Read the model definition and answer for the solid it produces. Units are mm, in the model's axes. Coordinates: 2 decimals unless noted, no trailing zeros. Write each loop counter-clockwise with the first axis right and the second up, starting at its lowest first coordinate (ties: lowest second). Pieces come first, ordered by that corner, then holes.
(1) Given pin 1 (10 mm diameter, centred on x = 1, z = -48.5, fed in from -Y); pin 2 (6 mm diameter, centred on y = 0, z = -180, fed in from +X); pin 3 (8 mm diameter, centred on x = -6, z = -57.5, fed in from -Y); pin 4 (10 mm diameter, centred on x = -8.5, z = -108, fed in from +Y), each flat-ended and moving along its own axis, determine where each tip first touches the part or whether it passes through.
(2) Section D-D on x = 23 is taken. Write down the section's boundary in (y, z), then the cut area to 3 significant figures.
(3) Section C-C on y = 23 is taken. Write down the section's boundary in (x, z).
(4) Find the intervals of material crossed by probe 1 along X at (y, z) = (-25, 6); probe 2 along Y at (x, z) = (25.6, 0); probe 3 along Y at (x, z) = (25.55, -180), in increasing order.
(5) Section B-B on y = 0 is taken. Write down the section's boundary in (x, z), then the cut area to 3 significant figures.
(6) Section A-A on z = 0 is taken. Write down the section's boundary in (x, y), then the cut area to 4 significant figures.
(7) The mould has two halves that part along Z. Classify faces 1 (the flat face through (0.364, -21.656, -93.869)), 2 (the flat face through (-25, 0, -56)), 3 (the flat face through (0.35, -21.12, -88.62)), 4 (the cylindrical face through (25.493, -0.751, -177.615)): +Z half, -Z half, draft (parallel to the pull), parting line (faces both ways), or undercut.
from build123d import *

# Parameters (mm, degrees)
SKETCH1_R           = 5
SKETCH1_R_2         = 2.5
BOSS_EXTRUDE1_DEPTH = 26
CUT_EXTRUDE1_DEPTH  = 25


with BuildPart() as part:
    # Sketch1 → Boss-Extrude1 (new, symmetric)
    with BuildSketch(Plane(origin=(0, 0, 0), x_dir=(0, 0, -1), z_dir=(1, 0, 0))):
        with BuildLine():
            Line((5.291523763, 29.529642332), (180, 14))
            ThreePointArc((180, 14), (194, 0), (180, -14))
            Line((180, -14), (5.291523763, -29.529642332))
            ThreePointArc((5.291523763, -29.529642332), (-30, 0), (5.291523763, 29.529642332))
        make_face()
        with Locations(Location((0, 0, 0), (0, 0, 180))):
            Circle(SKETCH1_R, mode=Mode.SUBTRACT)
        with Locations(Location((180, 0, 0), (0, 0, 180))):
            Circle(SKETCH1_R_2, mode=Mode.SUBTRACT)
    extrude(amount=BOSS_EXTRUDE1_DEPTH, both=True)

    # Sketch2 → Cut-Extrude1 (cut, symmetric)
    with BuildSketch(Plane(origin=(0, 0, 0), x_dir=(0, 0, -1), z_dir=(1, 0, 0))):
        with BuildLine():
            Line((5.291523763, -29.529642332), (5.114444182, -28.541439895))
            Line((5.114444182, -28.541439895), (174.506520913, -13.484366408))
            Line((174.506520913, -13.484366408), (174.595060704, -14.480439049))
            Line((174.595060704, -14.480439049), (180, -14))
            ThreePointArc((180, -14), (194, 0), (180, 14))
            Line((180, 14), (5.291523763, 29.529642332))
            ThreePointArc((5.291523763, 29.529642332), (-30, 0), (5.291523763, -29.529642332))
        make_face()
    extrude(amount=CUT_EXTRUDE1_DEPTH, both=True, mode=Mode.SUBTRACT)


solid = part.part
Response:
1. pin 1: stops at y = -26.13
1. pin 2: stops at x = 26
1. pin 3: stops at y = -25.24
1. pin 4: stops at y = -18.95
2. outline: (-29.53, -5.29) - (-14.48, -174.6) - (-13.48, -174.51) - (-28.54, -5.11) - close
2. area: 170 mm2
3. outline: (-26, -78.75) - (-25, -78.75) - (-25, 19.26) - (-26, 19.26) - close; (25, -78.75) - (26, -78.75) - (26, 19.26) - (25, 19.26) - close
4. probe 1: x = -26 to -25, 25 to 26
4. probe 2: y = -30 to -5, 5 to 30
4. probe 3: y = -14 to -2.5, 2.5 to 14
5. outline: (-26, -194) - (-25, -194) - (-25, -182.5) - (-26, -182.5) - close; (-26, -177.5) - (-25, -177.5) - (-25, -5) - (-26, -5) - close; (-26, 5) - (-25, 5) - (-25, 30) - (-26, 30) - close; (25, -194) - (26, -194) - (26, -182.5) - (25, -182.5) - close; (25, -177.5) - (26, -177.5) - (26, -5) - (25, -5) - close; (25, 5) - (26, 5) - (26, 30) - (25, 30) - close
5. area: 418 mm2
6. outline: (-26, -30) - (-25, -30) - (-25, -5) - (-26, -5) - close; (-26, 5) - (-25, 5) - (-25, 30) - (-26, 30) - close; (25, -30) - (26, -30) - (26, -5) - (25, -5) - close; (25, 5) - (26, 5) - (26, 30) - (25, 30) - close
6. area: 100.0 mm2
7. face 1: -Z half
7. face 2: draft
7. face 3: +Z half
7. face 4: undercut
